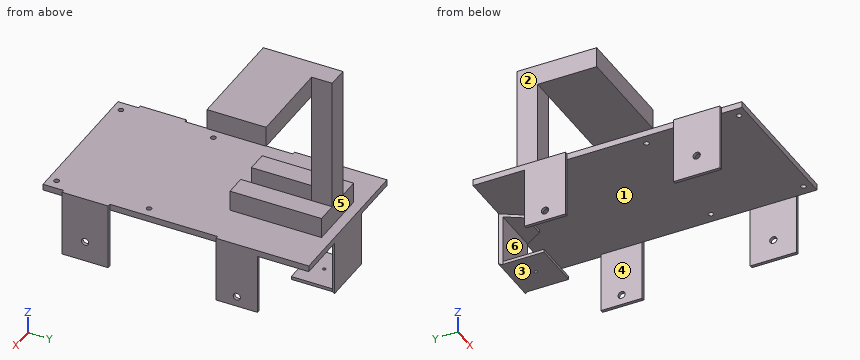
Autodesk Inventor part; units mm, degrees
ref_plane "Work Plane1" through (75.5, 0, 14.5) normal (1, 0, 0) x (0, 0, -1)
ref_plane "Work Plane2" through (75.5, 250, 14.5) normal (1, 0, 0) x (0, 0, -1)
ref_plane "Work Plane3" through (85.5, 117.5, 14.5) normal (-1, 0, 0) x (0, 0, 1)
sketch "Sketch2" plane through (0, 0, 0) normal (0, 1, 0) x (-1, 0, 0)
  line L0 (-25.5, 14.5) -> (-5.5, 14.5)
  line L1 (-5.5, 14.5) -> (-5.5, -5.5)
  line L2 (-5.5, -5.5) -> (-25.5, -5.5)
  line L3 (-25.5, -5.5) -> (-25.5, 14.5)
  line L4 (-25.5, 14.5) -> (-5.5, -5.5) construction
  line L5 (-5.5, 14.5) -> (-25.5, -5.5) construction
  point P0 (0, 0)
  point P1 (-15.5, 4.5)
  dimension "d0" = 20
  dimension "d1" = 20
extrude "Extrusion1" add sketch "Sketch2" along normal blind 210
sketch "Sketch3" plane through (25.5, 0, 14.5) normal (1, 0, 0) x (0, 0, -1)
  line L0 (20, 0) -> (20, 210)
  line L1 (0, 137.5) -> (20, 137.5)
  line L2 (20, 137.5) -> (20, 117.5)
  line L3 (20, 117.5) -> (0, 117.5)
  line L4 (0, 117.5) -> (0, 137.5)
  line L5 (0, 137.5) -> (20, 117.5) construction
  line L6 (20, 137.5) -> (0, 117.5) construction
  point P0 (14.5, 0)
  point P1 (10, 127.5)
  dimension "d4" = 20
extrude "Extrusion2" add sketch "Sketch3" along normal blind 100
ref_plane "Work Plane1" through (75.5, 0, 14.5) normal (1, 0, 0) x (0, 0, -1)
mirror "Mirror1" about plane through (75.5, 0, 14.5) normal (1, 0, 0) of "Extrusion1"
sketch "Sketch4" plane through (5.5, 0, 14.5) normal (0, 0, 1) x (1, 0, 0)
  line L0 (60, 250) -> (80, 250)
  line L1 (80, 250) -> (80, 230)
  line L2 (80, 230) -> (60, 230)
  line L3 (60, 230) -> (60, 250)
  line L4 (60, 250) -> (80, 230) construction
  line L5 (80, 250) -> (60, 230) construction
  point P0 (-5.5, 0)
  point P1 (20, 112.5)
  point P2 (70, 240)
extrude "Extrusion3" add sketch "Sketch4" along normal blind 150
sketch "Sketch11" plane through (5.5, 0, 14.5) normal (0, 0, 1) x (1, 0, 0)
  circle A0 centre (10, 8) radius 2.5
  circle A1 centre (10, 98) radius 2.5
  circle A2 centre (130, 8) radius 2.5
  circle A3 centre (130, 98) radius 2.5
  point P0 (-5.5, 0)
  dimension "d25" = 5
  dimension "d28" = 90
  dimension "d31" = 120
  dimension "d39" = 120
extrude "Extrusion10" cut sketch "Sketch11" against normal blind 36
sketch "Sketch13" plane through (5.5, 0, 14.5) normal (0, 0, 1) x (1, 0, 0)
  circle A0 centre (130, 8) radius 2.5
  circle A1 centre (10, 8) radius 2.5
  circle A2 centre (10, 98) radius 2.5
  circle A3 centre (130, 98) radius 2.5
  line L0 (0, 110) -> (150, 110)
  line L1 (0, 110) -> (0, 0)
  line L2 (0, 0) -> (150, 0)
  line L3 (150, 0) -> (150, 110)
  line L4 (0, 110) -> (0, 55)
  line L5 (0, 55) -> (150, 55)
  point P0 (-5.5, 0)
  dimension "d36" = 55
sketch "Sketch14" plane through (145.5, 0, 14.5) normal (1, 0, 0) x (0, 0, -1)
  line L0 (0, 20) -> (65, 20)
  line L1 (65, 20) -> (65, 65)
  line L2 (65, 65) -> (0, 65)
  line L3 (0, 65) -> (0, 20)
  circle A0 centre (45, 42.5) radius 3.5
  dimension "d44" = 7
  dimension "d45" = 20
  dimension "d94" = 22.5
ref_plane "Work Plane2" through (75.5, 250, 14.5) normal (1, 0, 0) x (0, 0, -1)
extrude "Extrusion12" add sketch "Sketch14" along normal blind 3
mirror "Mirror3" about plane through (75.5, 250, 14.5) normal (1, 0, 0) of "Extrusion12"
sketch "Sketch15" plane through (5.5, 0, 14.5) normal (0, 0, 1) x (1, 0, 0)
  line L0 (0, 0) -> (0, 20)
  line L1 (20, 0) -> (0, 0)
  line L2 (0, 0) -> (140, 0)
  line L3 (140, 0) -> (140, 110)
  line L4 (0, 110) -> (0, 0)
  line L5 (0, 110) -> (140, 110)
  circle A0 centre (10, 98) radius 2.5
  circle A1 centre (10, 8) radius 2.5
  circle A2 centre (130, 98) radius 2.5
  circle A3 centre (130, 8) radius 2.5
  point P0 (-5.5, 0)
sketch "Sketch18" plane through (5.5, 210, -5.5) normal (-1, 0, 0) x (0, 0, 1)
  line L0 (20, 0) -> (-45, 0)
  line L1 (-45, 0) -> (-45, -40)
  line L2 (-45, -40) -> (20, -40)
  line L3 (20, -40) -> (20, 0)
  point P0 (5.5, -210)
  point P1 (-35, -20)
  dimension "d51" = 65
  dimension "d92" = 10
  dimension "d93" = 20
extrude "Extrusion13" add sketch "Sketch18" along normal blind 3
mirror "Mirror4" about plane through (75.5, 250, 14.5) normal (1, 0, 0) of "Extrusion13"
sketch "Sketch19" plane through (2.5, 210, -5.5) normal (-1, 0, 0) x (0, 0, 1)
  line L0 (-45, 0) -> (-45, -40)
  circle A0 centre (-35, -20) radius 3.5
  point P0 (5.5, -210)
  dimension "d54" = 7
  dimension "d55" = 10
extrude "Extrusion14" cut sketch "Sketch19" against normal through all
sketch "Sketch20" plane through (25.5, 0, 14.5) normal (1, 0, 0) x (0, 0, -1)
  line L0 (20, 117.5) -> (0, 117.5)
  line L1 (0, 0) -> (0, 117.5)
  line L2 (20, 0) -> (0, 0)
  line L3 (0, 0) -> (0, 117.5)
  line L4 (6, 117.5) -> (6, 0)
  line L5 (0, 137.5) -> (0, 210)
  line L6 (0, 210) -> (20, 210)
  line L7 (6, 210) -> (6, 137.5)
  line L8 (6, 137.5) -> (0, 137.5)
  point P0 (14.5, 0)
extrude "Extrusion15" add sketch "Sketch20" along normal up to next
sketch "Sketch21" plane through (0, 0, 0) normal (0, -1, 0) x (1, 0, 0)
  line L0 (145.5, 14.5) -> (145.5, -5.5)
  line L1 (5.5, -5.5) -> (145.5, -5.5)
  line L2 (145.5, -5.5) -> (145.5, 8.5)
  line L3 (145.5, 8.5) -> (5.5, 8.5)
  line L4 (5.5, 8.5) -> (5.5, -5.5)
  point P0 (0, 0)
extrude "Extrusion16" cut sketch "Sketch21" against normal through all
sketch "Sketch22" plane through (145.5, 210, 8.5) normal (0, 0, -1) x (-1, 0, 0)
  line L0 (0, 0) -> (140, 0)
  line L1 (70, 50) -> (45, 50)
  line L2 (70, 50) -> (95, 50)
  line L3 (70, 30) -> (82.5, 30)
  line L4 (82.5, 30) -> (70, 30)
  line L5 (82.5, 30) -> (95, 50)
  line L6 (57.5, 30) -> (70, 30)
  line L7 (57.5, 30) -> (45, 50)
  point P0 (145.5, -210)
  point P1 (70, 50)
extrude "Extrusion17" add sketch "Sketch22" along normal blind 3
sketch "Sketch25" plane through (0, 210, 0) normal (0, 1, 0) x (1, 0, 0)
  line L0 (145.5, -8.5) -> (5.5, -8.5)
  line L1 (148.5, -14.5) -> (148.5, 50.5)
  line L2 (2.5, -14.5) -> (148.5, -14.5)
  line L3 (148.5, -14.5) -> (148.5, -8.5)
  line L4 (148.5, -8.5) -> (2.5, -8.5)
  line L5 (2.5, -8.5) -> (2.5, -14.5)
  point P0 (100.5, -8.5)
  point P1 (0, 0)
extrude "Extrusion20" add sketch "Sketch25" along normal blind 50
sketch "Sketch26" plane through (145.5, 210, 5.5) normal (0, 0, -1) x (-1, 0, 0)
  line L0 (95, 50) -> (45, 50)
  line L1 (45, 50) -> (57.5, 30)
  line L2 (57.5, 30) -> (82.5, 30)
  line L3 (82.5, 30) -> (95, 50)
  line L4 (46.875, 47) -> (93.125, 47)
  point P0 (145.5, -210)
  dimension "d73" = 3
extrude "Extrusion21" add sketch "Sketch26" along normal blind 50 contours L3 L4 L1 L0
sketch "Sketch27" plane through (52.375, 257, 5.5) normal (0, -1, 0) x (1, 0, 0)
  line L0 (46.25, 0) -> (46.25, -50)
  line L1 (0, -50) -> (46.25, -50)
  line L2 (46.25, -50) -> (46.25, -47)
  line L3 (46.25, -47) -> (0, -47)
  line L4 (0, -47) -> (0, -50)
  point P0 (-52.375, -5.5)
extrude "Extrusion22" add sketch "Sketch27" along normal blind 40
sketch "Sketch28" plane through (5.5, 0, 14.5) normal (0, 0, 1) x (1, 0, 0)
  line L0 (60, 250) -> (40, 250)
  line L1 (40, 250) -> (40, 161)
  line L2 (40, 161) -> (60, 161)
  line L3 (60, 161) -> (60, 250)
  line L4 (80, 250) -> (100, 250)
  line L5 (100, 250) -> (100, 161)
  line L6 (100, 161) -> (80, 161)
  line L7 (80, 161) -> (80, 250)
  point P0 (-5.5, 0)
extrude "Extrusion23" add sketch "Sketch28" along normal blind 20
ref_plane "Work Plane3" through (85.5, 117.5, 14.5) normal (-1, 0, 0) x (0, 0, 1)
sketch "Sketch29" plane through (85.5, 117.5, 14.5) normal (-1, 0, 0) x (0, 0, 1)
  line L0 (130, 112.5) -> (150, 112.5)
  line L1 (130, 112.5) -> (130, 55)
  line L2 (130, 55) -> (150, 55)
  line L3 (150, 55) -> (150, 112.5)
  point P0 (-14.5, -117.5)
extrude "Extrusion24" add sketch "Sketch29" along normal blind 20
ref_plane "Work Plane4" through (170.5, 117.5, 14.5) normal (1, 0, 0) x (0, 0, -1)
sketch "Sketch32" plane through (85.5, 230, 34.5) normal (1, 0, 0) x (0, 0, -1)
  line L0 (-130, -57.5) -> (-130, 20)
  line L1 (-110, -57.5) -> (-130, -57.5)
  line L2 (-110, 0) -> (-110, -57.5)
  line L3 (0, 0) -> (-110, 0)
  line L4 (-130, 0) -> (-110, 0)
  point P0 (34.5, -230)
extrude "Extrusion26" add sketch "Sketch32" along normal blind 85
sketch "Sketch34" plane through (145.5, 210, -44.5) normal (0, 0, -1) x (-1, 0, 0)
  circle A0 centre (70, 27) radius 1.5
  point P0 (145.5, -210)
  dimension "d89" = 3
extrude "Extrusion27" cut sketch "Sketch34" against normal blind 5
properties part number "robot chasis"
Read the model definition and answer for the solid it produces. Units are mm, in the model's axes. Face numbers are marked on the shaded views. A direction names the side the tool comes from. Coordinates: 2 decimals unless noted, no trailing zeros. Write each loop counter-clockwise with the first axis right and the second up, starting at its lowest first coordinate (ties: lowest second). Pieces come first, ordered by that corner, then holes. Notation, with made-up numbers: M -21,49.5 L 16,49.5 A18 cw 16,81.5 Z; hole C 87.25,55.25 d10. An arc over 180 degrees is marked long. Use a Markdown table: item, result.
Q1. The part is cut by section B-B, the plane y = 42.5. Write down the section's boundary in (x, z).
Answer block:
| item | result |
|---|---|
| outline | M 2.5,-50.5 L 5.5,-50.5 L 5.5,-34 L 2.5,-34 Z; M 2.5,-27 L 5.5,-27 L 5.5,8.5 L 145.5,8.5 L 145.5,-27 L 148.5,-27 L 148.5,14.5 L 2.5,14.5 Z; M 145.5,-50.5 L 148.5,-50.5 L 148.5,-34 L 145.5,-34 Z |
Q2. Which of the six approach directions +Z, -Z, +X, -X, +Y, -Y give full straight-line access (tool end or side, diameter ignored) to the marked faces 4, 5 and 6?
Answer block:
| item | result |
|---|---|
| face 4 | -Z, +Y, -Y |
| face 5 | +Z, +X, -X, +Y |
| face 6 | +X, -X, -Y |
Q3. The part is cut by section C-C, the plane z = 76. Write down the section's boundary in (x, y).
Answer block:
| item | result |
|---|---|
| outline | M 65.5,230 L 85.5,230 L 85.5,250 L 65.5,250 Z |
Q4. The part is cut by section A-A, the plane x = 120. Write down the section's boundary in (y, z), then the cut area to 3 significant figures.
Answer block:
| item | result |
|---|---|
| outline | M 0,8.5 L 260,8.5 L 260,14.5 L 0,14.5 Z; M 172.5,144.5 L 230,144.5 L 230,164.5 L 172.5,164.5 Z |
| area | 2,710 mm2 |
Q5. Straight lines are drawn through the part: L1, parallel to Y at x = 147, z = -40; L2, parallel to Y at x = 135.5, z = 12.55; L3, parallel to Z at x = 147, y = 42. For each, find the intervals that lie inside material, in ascending order. Write a range as [from, to].
Answer block:
| item | result |
|---|---|
| L1 | y = [20, 65], [170, 186.54], [193.46, 210] |
| L2 | y = [0, 5.5], [10.5, 95.5], [100.5, 260] |
| L3 | z = [-50.5, -33.96], [-27.04, 14.5] |
Q6. Each of these flat-tipped pins is pushed along its axis until it touches: pin 1 Ø1.5 at (x, z) = (56, -15.5) entering from -Y; pin 2 Ø6 at (y, z) = (225.5, 20) entering from -X; pin 3 Ø1.8 at (y, z) = (7, 10.5) entering from -X. Where does it stop, or does it pass through?
Answer block:
| item | result |
|---|---|
| pin 1 | stops at y = 257 |
| pin 2 | stops at x = 45.5 |
| pin 3 | stops at x = 5.5 |
Q7. The part is cut by section D-D, the plane y = 142. Write down the section's boundary in (x, z).
Answer block:
| item | result |
|---|---|
| outline | M 5.5,8.5 L 145.5,8.5 L 145.5,14.5 L 5.5,14.5 Z |
Q8. Determine the mould class of the marked faces 1, 2 and 3 for opening direction X: released by +X, released by -X, zero draft, split by the parting line, or undercut.
Answer block:
| item | result |
|---|---|
| face 1 | undercut |
| face 2 | released by -X |
| face 3 | zero draft |
